```python
from build123d import *

# Parameters (mm, degrees)
BASPROSKE_W        = 10
BASPROSKE_H        = 8
TOOTHCUT_DEPTH     = 16.099668871
TEETHCUTS_COUNT    = 14
TEETHCUTS_ANGLE    = 334.285714286
BORSKE_R           = 1.5
BORE_DEPTH         = 50.0000508
CUT_EXTRUDE1_DEPTH = 4


with BuildPart() as part:
    # BasProSke → Base-Revolve (revolve)
    with BuildSketch(Plane(origin=(0, 0, 0), x_dir=(1, 0, 0), z_dir=(0, 1, 0)), mode=Mode.PRIVATE) as base_revolve_sk:
        with Locations((5, 4)):
            Rectangle(BASPROSKE_W, BASPROSKE_H)
    revolve(base_revolve_sk.sketch.rotate(Axis((-10, 0, 0), (1, 0, 0)), 180), axis=Axis((-10, 0, 0), (1, 0, 0)))

    # TooCutSke → ToothCut (cut, through all)
    with BuildSketch(Plane(origin=(0, 0, 0), x_dir=(0, 0, -1), z_dir=(1, 0, 0))):
        with BuildLine():
            ThreePointArc((0.540393256, 5.723545765), (0, 5.749), (-0.540393256, 5.723545765))
            ThreePointArc((-0.540393256, 5.723545765), (-0.832220085, 6.912663993), (-1.603550271, 7.863566092))
            ThreePointArc((-1.603550271, 7.863566092), (0, 8.0254), (1.603550271, 7.863566092))
            ThreePointArc((1.603550271, 7.863566092), (0.832220085, 6.912663993), (0.540393256, 5.723545765))
        make_face()
    toothcut = extrude(amount=TOOTHCUT_DEPTH, mode=Mode.SUBTRACT)

    # TeethCuts: ToothCut ×14 about axis
    teethcuts_axis = Axis((-10, 0, 0), (1, 0, 0))
    for i in range(1, TEETHCUTS_COUNT):
        add(toothcut.rotate(teethcuts_axis, i * TEETHCUTS_ANGLE / (TEETHCUTS_COUNT - 1)), mode=Mode.SUBTRACT)

    # BorSke → Bore (cut, symmetric)
    with BuildSketch(Plane(origin=(0, 0, 0), x_dir=(0, 0, -1), z_dir=(1, 0, 0))):
        with Locations(Location((0, 0, 0), (0, 0, 180))):
            Circle(BORSKE_R)
    extrude(amount=BORE_DEPTH, both=True, mode=Mode.SUBTRACT)

    # Sketch1 → Cut-Extrude1 (cut)
    with BuildSketch(Plane.ZY):
        Polygon((0.37552517, 2.972587809), (0, 2.7), (-0.37552517, 2.972587809), (-0.671462695, 2.615174535), (-1.102979883, 2.785809184), (-1.30073492, 2.366028036), (-1.761130314, 2.423987923), (-1.848277186, 1.968215294), (-2.308622449, 1.909858586), (-2.279685399, 1.446732346), (-2.711055346, 1.27572581), (-2.567852594, 0.834345885), (-2.943142665, 0.56143449), (-2.694672167, 0.169534403), (-2.990301506, -0.188133824), (-2.652175577, -0.505929549), (-2.849568706, -0.925880998), (-2.443033042, -1.149604087), (-2.529787024, -1.605451664), (-2.080385755, -1.721044772), (-2.05104952, -2.184145897), (-1.587020181, -2.184345885), (-1.44343703, -2.625602211), (-0.993936292, -2.510396512), (-0.745128084, -2.902082282), (-0.338399731, -2.678709694), (0, -2.99621385), (0.338399731, -2.678709694), (0.745128084, -2.902082282), (0.993936292, -2.510396512), (1.44343703, -2.625602211), (1.587020181, -2.184345885), (2.05104952, -2.184145897), (2.080385755, -1.721044772), (2.529787024, -1.605451664), (2.443033042, -1.149604087), (2.849568706, -0.925880998), (2.652175577, -0.505929549), (2.990301506, -0.188133824), (2.694672167, 0.169534403), (2.943142665, 0.56143449), (2.567852594, 0.834345885), (2.711055346, 1.27572581), (2.279685399, 1.446732346), (2.308622449, 1.909858586), (1.848277186, 1.968215294), (1.761130314, 2.423987923), (1.30073492, 2.366028036), (1.102979883, 2.785809184), (0.671462695, 2.615174535), align=None)
    extrude(amount=-CUT_EXTRUDE1_DEPTH, mode=Mode.SUBTRACT)


solid = part.part
```
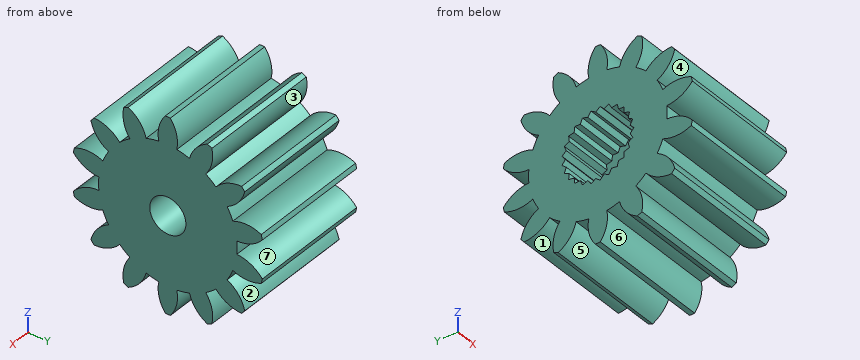
Source: CAD feature listing. Evaluate the final solid. Frame: model axes, mm. Face numbers are marked on the shaded views. A direction names the side the tool comes from. Round coordinates to 2 decimals unless told otherwise and drop trailing zeros. Loops run counter-clockwise (first coordinate to the right, second up) from the corner with the lowest first, then second, coordinate; pieces in that order, holes last.
(1) Pull-direction query (Y, two-part tool) for the marked faces 1, 2, 3 and 4; classes: +Y half, -Y half, draft (parallel to the pull), parting line (faces both ways), or undercut.
From the geometry:
face 1: undercut
face 2: +Y half
face 3: undercut
face 4: -Y half
(2) Contact query for flat-ended pins moving along their axis: pin 1 Ø3 at (x, y) = (4.5, -3.5) entering from -Z; pin 2 Ø4 at (x, y) = (4, -3) entering from +Z; pin 3 Ø1.5 at (x, y) = (8, 2) entering from +Z. Output: stop coordinate, or through.
From the geometry:
pin 1: stops at z = -7.3
pin 2: stops at z = 7.3
pin 3: stops at z = 6.95
(3) Section query A-A (y = 7). Output: boundary loops of the cut face in (x, z).
From the geometry:
outline: (0, -2.21) - (10, -2.21) - (10, -0.88) - (0, -0.88) - close; (0, 0.88) - (10, 0.88) - (10, 2.21) - (0, 2.21) - close
(4) Access query for the marked faces 5, 6 and 7. Directions: +Z, -Z, +X, -X, +Y, -Y. A direction counts if a zero-diameter tool reaches every point of the face in a straight line with its end or side. Return the directions, or none.
From the geometry:
face 5: -Z, +X, -X
face 6: +X, -X
face 7: +X, -X, +Y
(5) Material intervals for probe 1 along Y at (x, z) = (5.6, 0); probe 2 along Y at (x, z) = (8, -6.5); probe 3 along Y at (x, z) = (4.5, -5.75), sorted ascending.
From the geometry:
probe 1: y = -5.75 to -1.5, 1.5 to 5.75
probe 2: y = -3.72 to -2.31, -0.8 to 0.8, 2.31 to 3.72
probe 3: y = -3.62 to -1.89, -0.76 to 0.76, 1.89 to 3.62
